Autodesk Inventor part; units mm, degrees
ref_plane "YZ Plane" through (0, 0, 0) normal (1, 0, 0) x (0, 1, 0)
ref_plane "XZ Plane" through (0, 0, 0) normal (0, 1, 0) x (-1, 0, 0)
ref_plane "XY Plane" through (0, 0, 0) normal (0, 0, 1) x (1, 0, 0)
sketch "Sketch1" plane through (0, 0, 0) normal (0, 0, 1) x (1, 0, 0)
  line L0 (0, 0) -> (25.4, 0)
  line L1 (25.4, 0) -> (25.4, 50.8)
  line L2 (25.4, 50.8) -> (0, 50.8)
  line L3 (0, 50.8) -> (0, 0)
  line L4 (3.175, 3.175) -> (22.225, 3.175)
  line L5 (22.225, 3.175) -> (22.225, 47.625)
  line L6 (22.225, 47.625) -> (3.175, 47.625)
  line L7 (3.175, 47.625) -> (3.175, 3.175)
  dimension "d0" = 25.4
  dimension "d1" = 50.8
  dimension "d2" = 19.05
  dimension "d3" = 44.45
  dimension "d4" = 3.175
  dimension "d5" = 3.175
extrude "Extrusion1" add sketch "Sketch1" along normal blind 711.2
sketch "Sketch9" plane through (0, 50.8, 0) normal (0, 1, 0) x (1, 0, 0)
  line L0 (25.4, 0) -> (0, 0)
  line L1 (0, 0) -> (0, -711.2)
  line L2 (25.4, -711.2) -> (0, -711.2)
  line L3 (25.4, 0) -> (25.4, -711.2)
  point P0 (12.7, -704.85)
  point P1 (12.7, -679.45)
  point P2 (12.7, -203.2)
  point P3 (12.7, -177.8)
  dimension "d75" = 6.35
  dimension "d76" = 12.7
  dimension "d77" = 12.7
  dimension "d78" = 31.75
  dimension "d79" = 12.7
  dimension "d80" = 12.7
  dimension "d81" = 508
  dimension "d82" = 533.4
hole "Hole6" at (12.7, 50.8, 704.85) at (12.7, 50.8, 679.45) at (12.7, 50.8, 203.2) at (12.7, 50.8, 177.8) direction (0, -1, 0) diameter 6.35 end through all
sketch "Sketch10" plane through (0, 0, 0) normal (-1, 0, 0) x (0, 0, 1)
  line L0 (0, 50.8) -> (0, 0)
  line L1 (0, 0) -> (711.2, 0)
  line L2 (711.2, 50.8) -> (711.2, 0)
  line L3 (0, 50.8) -> (711.2, 50.8)
  point P0 (704.85, 12.7)
  point P1 (679.45, 12.7)
  point P2 (273.05, 12.7)
  point P3 (247.65, 12.7)
  point P4 (222.25, 12.7)
  point P5 (654.05, 12.7)
  dimension "d90" = 6.35
  dimension "d91" = 12.7
  dimension "d92" = 12.7
  dimension "d93" = 31.75
  dimension "d94" = 12.7
  dimension "d95" = 12.7
  dimension "d96" = 438.15
  dimension "d97" = 463.55
  dimension "d130" = 12.7
  dimension "d131" = 488.95
  dimension "d132" = 12.7
  dimension "d133" = 57.15
sketch "Sketch11" plane through (0, 0, 0) normal (-1, 0, 0) x (0, 0, 1)
  line L0 (0, 50.8) -> (0, 0)
  line L1 (0, 0) -> (711.2, 0)
  line L2 (711.2, 50.8) -> (711.2, 0)
  line L3 (0, 50.8) -> (711.2, 50.8)
  point P0 (190.5, 25.4)
  dimension "d105" = 25.4
  dimension "d129" = 520.7
hole "Hole8" at (0, 25.4, 190.5) direction (1, 0, 0) diameter 19.05 end through all
hole "Hole10" at (0, 12.7, 704.85) at (0, 12.7, 679.45) at (0, 12.7, 273.05) at (0, 12.7, 247.65) at (0, 12.7, 222.25) at (0, 12.7, 654.05) direction (1, 0, 0) diameter 6.35 end through all
sketch "Sketch13" plane through (25.4, 0, 0) normal (1, 0, 0) x (0, 0, -1)
  circle A0 centre (-222.25, 12.7) radius 3.175
  circle A1 centre (-273.05, 12.7) radius 3.175
  circle A2 centre (-704.85, 12.7) radius 3.175
  circle A3 centre (-679.45, 12.7) radius 3.175
  circle A4 centre (-247.65, 12.7) radius 3.175
  circle A5 centre (-654.05, 12.7) radius 3.175
  circle A6 centre (-190.5, 25.4) radius 9.525
  line L0 (0, 0) -> (0, 50.8)
  line L1 (0, 50.8) -> (-711.2, 50.8)
  line L2 (-711.2, 0) -> (-711.2, 50.8)
  line L3 (0, 0) -> (-711.2, 0)
  point P0 (-247.65, 38.1)
  point P1 (-222.25, 38.1)
  dimension "d141" = 12.7
  dimension "d142" = 12.7
  dimension "d143" = 463.55
  dimension "d144" = 488.95
hole "Hole11" at (25.4, 38.1, 247.65) at (25.4, 38.1, 222.25) direction (-1, 0, 0) diameter 6.35 end through all
sketch "Sketch14" plane through (25.4, 0, 0) normal (1, 0, 0) x (0, 0, -1)
  circle A0 centre (-247.65, 38.1) radius 3.175
  circle A1 centre (-222.25, 38.1) radius 3.175
  circle A2 centre (-222.25, 12.7) radius 3.175
  circle A3 centre (-273.05, 12.7) radius 3.175
  circle A4 centre (-704.85, 12.7) radius 3.175
  circle A5 centre (-679.45, 12.7) radius 3.175
  circle A6 centre (-247.65, 12.7) radius 3.175
  circle A7 centre (-654.05, 12.7) radius 3.175
  circle A8 centre (-190.5, 25.4) radius 9.525
  line L0 (0, 0) -> (0, 50.8)
  line L1 (0, 50.8) -> (-711.2, 50.8)
  line L2 (-711.2, 0) -> (-711.2, 50.8)
  line L3 (0, 0) -> (-711.2, 0)
  line L4 (-38.1, 25.4) -> (-17.4778, 37.3062) construction
  line L5 (-38.1, 25.4) -> (-14.2875, 25.4) construction
  line L6 (-38.1, 25.4) -> (-17.4778, 13.4938) construction
  line L7 (-38.1, 25.4) -> (-14.2875, 25.4) construction
  line L8 (-38.1, 25.4) -> (-58.7222, 37.3063) construction
  line L9 (-38.1, 25.4) -> (-14.2875, 25.4) construction
  line L10 (-38.1, 25.4) -> (-58.7222, 13.4938) construction
  line L11 (-38.1, 25.4) -> (-14.2875, 25.4) construction
  circle A9 centre (-38.1, 25.4) radius 7.9375
  circle A10 centre (-58.7222, 37.3063) radius 2.54
  circle A11 centre (-58.7222, 13.4938) radius 2.54
  circle A12 centre (-17.4778, 13.4938) radius 2.54
  circle A13 centre (-17.4778, 37.3062) radius 2.54
  dimension "d152" = 38.1
  dimension "d153" = 25.4
  dimension "d154" = 23.8125
  dimension "d155" = 30
  dimension "d156" = 23.8125
  dimension "d157" = 30
  dimension "d158" = 23.8125
  dimension "d159" = 150
  dimension "d160" = 23.8125
  dimension "d161" = 150
  dimension "d162" = 15.875
  dimension "d163" = 5.08
  dimension "d164" = 5.08
  dimension "d165" = 5.08
  dimension "d166" = 5.08
extrude "Extrusion4" cut sketch "Sketch14" against normal blind 25.4 contours A9 | A10 | A11 | A12 | A13
properties part number "2x1"
Geometry: final body of the model. Coordinates: model frame, mm. A direction names the side the tool comes from. Give positions to 0.01 mm unless a question says otherwise; leave off trailing zeros. Order: outer loops, then holes, each group sorted by start corner. A loop starts at its lowest first (then second) coordinate and runs counter-clockwise, first axis right, second up. Notation, with made-up numbers: (75, 6.5) -> (96, 6.5) arc R30 cw to (96, 45.5) -> close; hole circle Ø7 at (-17.75, 73.5). An arc over 180 degrees is marked (long way). Put each result on its own line as item: value.
Q1. Section D-D, the plane z = 190.5. Return loops of the section in (x, y) (3 decimals), then the cut area to 3 significant figures.
Here are the results:
outline: (0, 0) -> (25.4, 0) -> (25.4, 15.875) -> (22.225, 15.875) -> (22.225, 3.175) -> (3.175, 3.175) -> (3.175, 15.875) -> (0, 15.875) -> close; (0, 34.925) -> (3.175, 34.925) -> (3.175, 47.625) -> (22.225, 47.625) -> (22.225, 34.925) -> (25.4, 34.925) -> (25.4, 50.8) -> (0, 50.8) -> close
area: 323 mm^2
Q2. Section B-B, the plane y = 25.4. Return loops of the section in (x, z) (1 decimal).
Here are the results:
outline: (0, 0) -> (3.2, 0) -> (3.2, 30.2) -> (0, 30.2) -> close; (0, 46) -> (3.2, 46) -> (3.2, 181) -> (0, 181) -> close; (0, 200) -> (3.2, 200) -> (3.2, 711.2) -> (0, 711.2) -> close; (22.2, 0) -> (25.4, 0) -> (25.4, 30.2) -> (22.2, 30.2) -> close; (22.2, 46) -> (25.4, 46) -> (25.4, 181) -> (22.2, 181) -> close; (22.2, 200) -> (25.4, 200) -> (25.4, 711.2) -> (22.2, 711.2) -> close
Q3. Section A-A, the plane z = 38.1. Return loops of the section in (x, y) (1 decimal).
Here are the results:
outline: (0, 0) -> (25.4, 0) -> (25.4, 17.5) -> (22.2, 17.5) -> (22.2, 3.2) -> (3.2, 3.2) -> (3.2, 17.5) -> (0, 17.5) -> close; (0, 33.3) -> (3.2, 33.3) -> (3.2, 47.6) -> (22.2, 47.6) -> (22.2, 33.3) -> (25.4, 33.3) -> (25.4, 50.8) -> (0, 50.8) -> close
Q4. Section C-C, the plane z = 335. Return loops of the section in (x, y) (3 decimals), then the cut area to 3 significant figures.
Here are the results:
outline: (0, 0) -> (25.4, 0) -> (25.4, 50.8) -> (0, 50.8) -> close; hole (3.175, 3.175) -> (22.225, 3.175) -> (22.225, 47.625) -> (3.175, 47.625) -> close
area: 444 mm^2
Q5. Draft query along X for faces 3 (the face through (2, 24, 0)), 4 (the face through (0, 26, 351)), 5 (the face through (13, 3.175, 351)). Return one class per face: released by +X, released by -X, zero draft, split by the parting line, or undercut.
Here are the results:
face 3: zero draft
face 4: released by -X
face 5: undercut
Q6. Material intervals for L1, parallel to Y at x = 24.3, z = 247.65 (3 decimals); L2, parallel to Z at x = 12.7, y = 49.05 (3 decimals); L3, parallel to X at y = 29.5, z = 394 (3 decimals), sorted ascending.
Here are the results:
L1: y = 0 to 9.525, 15.875 to 34.925, 41.275 to 50.8
L2: z = 0 to 174.625, 180.975 to 200.025, 206.375 to 676.275, 682.625 to 701.675, 708.025 to 711.2
L3: x = 0 to 3.175, 22.225 to 25.4
Q7. Reachability of faces 1 (the face through (22.225, 25, 351)), 2 (the face through (25.4, 25, 351)) from +Z, -Z, +X, -X, +Y, -Y: full face, straight path, thin tool, end or side. Return the list, or none.
Here are the results:
face 1: +Z, -Z
face 2: +Z, -Z, +X, +Y, -Y
Q8. Pin query (flat end, axial travel): pin 1 (10 mm diameter, centred on y = 11.5, z = 426.5, fed in from -X). Return the tip coordinate at first contact, or that it passes through.
Here are the results:
pin 1: stops at x = 0
